from build123d import *

# Parameters (mm, degrees)
SKETCH2_R          = 14.644408022
CUT_EXTRUDE1_DEPTH = 40


with BuildPart() as part:
    # Sketch1 → Revolve1 (revolve)
    with BuildSketch(Plane.XY, mode=Mode.PRIVATE) as revolve1_sk:
        Polygon((0, 0), (0, -25), (40, -25), (40, -30), (65.930548057, -30), (65.930548057, -25), (85.930548057, -25), (85.930548057, -20), (105.930548057, -20), (105.930548057, -15), (125.930548057, -15), (125.930548057, -10), (145.930548057, -10), (145.930548057, -5), (165.930548057, -5), (165.930548057, -2.5), (185.930548057, -2.5), (185.930548057, 0), align=None)
    revolve(revolve1_sk.sketch.rotate(Axis((0, 0, 0), (1, 0, 0)), 270), axis=Axis((0, 0, 0), (1, 0, 0)))  # turned: the seam where the file's is

    # Sketch2 → Cut-Extrude1 (cut)
    with BuildSketch(Plane.ZY):
        Circle(SKETCH2_R)
    extrude(amount=-CUT_EXTRUDE1_DEPTH, mode=Mode.SUBTRACT)


solid = part.part
Verification items for the finished model (mm, model axes). A direction names the side the tool comes from. Round coordinates to 2 decimals unless told otherwise and drop trailing zeros. Loops run counter-clockwise (first coordinate to the right, second up) from the corner with the lowest first, then second, coordinate; pieces in that order, holes last. Notation, with made-up numbers: (77.5, -4) - (134.5, -4) arc R13 ccw to (134.5, 17) - close; hole circle Ø7 at (78.25, 48). An arc over 180 degrees is marked (long way). Use a Markdown table: item, result. Add a question column.
1. Gauge pin test, flat ends, axial feed: pin 1 (2 mm diameter, centred on x = 94.5, z = 10, fed in from -Y); pin 2 (20 mm diameter, centred on y = 7.5, z = -1, fed in from +X); pin 3 (4 mm diameter, centred on x = 85.5, y = -14.5, fed in from -Z); pin 4 (18 mm diameter, centred on y = 3, z = -1.5, fed in from -X). Record the tip position at first contact, or that the pin passes through.
2. Section check C-C, the plane z = 7.5. Record the boundary of the cut face in (x, y), plus the area to 3 significant figures.
3. Release check for a two-part mould opening along Z. For faces 1 (the face through (136.07, 9.76, -2.17)), 2 (the face through (40, -25, 7)), 3 (the face through (19.72, -14.296, -3.175)) record: released by +Z, released by -Z, zero draft, split by the parting line, or undercut.
4. Thickness scan on probe 1 along Y at (x, z) = (13, 0); probe 2 along X at (y, z) = (-14, -6.5); probe 3 along X at (y, z) = (7, 25.5). Record the ranges inside material, lowest first. Write a range as [from, to].
5. Section check A-A, the plane x = 68.5. Record the boundary of the cut face in (y, z).
6. Access from +Z, -Z, +X, -X, +Y, -Y to the whole of each face (thin tool, end or side, straight path). Record for faces 4 (the face through (0, 11, -11)), 5 (the face through (20.28, -7.509, 23.846)), 6 (the face through (156.07, 4.88, -1.08)).
7. Section check B-B, the plane y = -7. Record the boundary of the cut face in (x, z) (1 decimal), plus the area to 3 significant figures.
8. Section check D-D, the plane x = 172.5. Record the boundary of the cut face in (y, z).
Checks:
| question | item | result |
|---|---|---|
| 1 | pin 1 | stops at y = -17.86 |
| 1 | pin 2 | stops at x = 185.93 |
| 1 | pin 3 | stops at z = -21.65 |
| 1 | pin 4 | stops at x = 40 |
| 2 | outline | (0, -23.85) - (40, -23.85) - (40, -29.05) - (65.93, -29.05) - (65.93, -23.85) - (85.93, -23.85) - (85.93, -18.54) - (105.93, -18.54) - (105.93, -12.99) - (125.93, -12.99) - (125.93, -6.61) - (145.93, -6.61) - (145.93, 6.61) - (125.93, 6.61) - (125.93, 12.99) - (105.93, 12.99) - (105.93, 18.54) - (85.93, 18.54) - (85.93, 23.85) - (65.93, 23.85) - (65.93, 29.05) - (40, 29.05) - (40, 23.85) - (0, 23.85) - (0, 12.58) - (40, 12.58) - (40, -12.58) - (0, -12.58) - close |
| 2 | area | 4,890 mm^2 |
| 3 | face 1 | split by the parting line |
| 3 | face 2 | zero draft |
| 3 | face 3 | undercut |
| 4 | probe 1 | y = [-25, -14.64], [14.64, 25] |
| 4 | probe 2 | x = [0, 105.93] |
| 4 | probe 3 | x = [40, 65.93] |
| 5 | outline | circle Ø50 at (0, 0) |
| 6 | face 4 | +Z, -Z, -X, +Y, -Y |
| 6 | face 5 | -X |
| 6 | face 6 | +X |
| 7 | outline | (0, -24) - (40, -24) - (40, -29.2) - (65.9, -29.2) - (65.9, -24) - (85.9, -24) - (85.9, -18.7) - (105.9, -18.7) - (105.9, -13.3) - (125.9, -13.3) - (125.9, -7.1) - (145.9, -7.1) - (145.9, 7.1) - (125.9, 7.1) - (125.9, 13.3) - (105.9, 13.3) - (105.9, 18.7) - (85.9, 18.7) - (85.9, 24) - (65.9, 24) - (65.9, 29.2) - (40, 29.2) - (40, 24) - (0, 24) - (0, 12.9) - (40, 12.9) - (40, -12.9) - (0, -12.9) - close |
| 7 | area | 4,930 mm^2 |
| 8 | outline | circle Ø5 at (0, 0) |
